from build123d import *

# Parameters (mm, degrees)
F0_W     = 215.9
F0_H     = 105
F1_DEPTH = 50.8
F2_R     = 1.5
F3_DEPTH = 5
F4_W     = 15
F4_H     = 101.8
F5_DEPTH = 40.8


with BuildPart() as f1:
    # F0 (on Top) → F1 (new body)
    with BuildSketch(Plane.XY):
        Rectangle(F0_W, F0_H)
    extrude(amount=F1_DEPTH)

    # F2 (on face) → F3 (cut)
    with BuildSketch(Plane.XY.offset(50.8)):
        with Locations((100.45, 42.5)):
            Circle(F2_R)
        with Locations((100.45, -42.5)):
            Circle(F2_R)
        with Locations((-77.95, -42.5)):
            Circle(F2_R)
        with Locations((-77.95, 42.5)):
            Circle(F2_R)
    extrude(amount=-F3_DEPTH, mode=Mode.SUBTRACT)

    # F4 (on face) → F5 (cut)
    with BuildSketch(Plane.XY.offset(50.8)):
        with Locations((-100.45, 0)):
            Rectangle(F4_W, F4_H)
    extrude(amount=-F5_DEPTH, mode=Mode.SUBTRACT)


solid = f1.part
The model under review builds one solid part; all positions refer to its coordinate system, in mm. A direction names the side the tool comes from. Coordinates: 2 decimals unless noted, no trailing zeros. Write each loop counter-clockwise with the first axis right and the second up, starting at its lowest first coordinate (ties: lowest second). Pieces come first, ordered by that corner, then holes. Notation, with made-up numbers: (67.5, -25.75) - (85.5, -25.75) arc R18 ccw to (85.5, -10.75) - close; hole circle Ø8 at (12.25, -10.75). An arc over 180 degrees is marked (long way). Answer as a JSON object with one key per item and string values. Group by question number.
1. Machinability: for faces 5 (the face through (22, 1, 50.8)), 6 (the face through (-101, 1, 10)), which of the approach directions +Z, -Z, +X, -X, +Y, -Y give a long, thin tool a straight path to every point of the face, cutting with its end or side? Answer none if there is none.
2. Add section B-B (y = -9). Give the boundary of the cut face in (x, z), plus the area to 3 significant figures.
3. Clearance check with flat-ended pins moving along their axes: pin 1 Ø2.5 at (x, y) = (-77.95, -42.5) entering from +Z; pin 2 Ø3.5 at (x, y) = (-77.5, -43) entering from +Z; pin 3 Ø8 at (y, z) = (19.5, 42) entering from -X; pin 4 Ø12 at (x, y) = (-100, -23.5) entering from +Z. State where each tip first meets the part, or that it passes through.
4. Add section A-A (z = 31). Give the boundary of the cut face in (x, y).
5. To check wall thickness, follow probe 1 along Y at (x, z) = (-77.95, 47.6); probe 2 along Y at (x, z) = (-94.5, 22); probe 3 along X at (y, z) = (-42, 49). State the ranges of each line that lie inside material, in increasing order.
6. Mouldability with a two-part tool opening along Y and no side actions: class faces 1 (the face through (-2, -52.5, 25)), 2 (the face through (-101, -50.9, 31)), 3 (the face through (-92.95, -1, 31)), 4 (the face through (-2, 1, 0)) as pulls with the +Y half, pulls with the -Y half, needs draft (parallel to the pull), parting line crosses it, or undercut.
Findings:
{
 "1": {"face 5": "+Z, +X, -X, +Y, -Y", "face 6": "+Z, -X"},
 "2": {"outline": "(-107.95, 0) - (107.95, 0) - (107.95, 50.8) - (-92.95, 50.8) - (-92.95, 10) - (-107.95, 10) - close", "area": "10,400 mm²"},
 "3": {"pin 1": "z = 45.8", "pin 2": "z = 50.8", "pin 3": "x = -92.95", "pin 4": "z = 10"},
 "4": {"outline": "(-107.95, -52.5) - (107.95, -52.5) - (107.95, 52.5) - (-107.95, 52.5) - (-107.95, 50.9) - (-92.95, 50.9) - (-92.95, -50.9) - (-107.95, -50.9) - close"},
 "5": {"probe 1": "-52.5 to -44, -41 to 41, 44 to 52.5", "probe 2": "-52.5 to -50.9, 50.9 to 52.5", "probe 3": "-92.95 to -79.36, -76.54 to 99.04, 101.86 to 107.95"},
 "6": {"face 1": "pulls with the -Y half", "face 2": "undercut", "face 3": "undercut", "face 4": "needs draft"}
}
